Input: part model. Units: mm. Frame: model coordinates. Face numbers are marked on the shaded views. Round coordinates to 2 decimals unless told otherwise and drop trailing zeros. Order: outer loops, then holes, each group sorted by start corner. A loop starts at its lowest first (then second) coordinate and runs counter-clockwise, first axis right, second up. Notation, with made-up numbers: (-38, 61.25) - (10, 61.25) arc R33 ccw to (10, 92.25) - close; hole circle Ø9 at (-19.5, 40.5). An arc over 180 degrees is marked (long way). One line per item, written item: value. Start each with the question number.
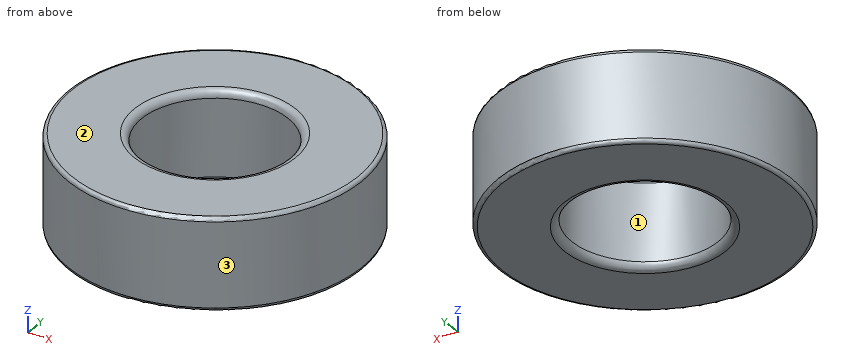
from build123d import *

# Parameters (mm, degrees)
BEARING_BOSS_EXTRUDE1_DEPTH      = 2.5
BEARING_BOSS_EXTRUDE1_DEPTH_BACK = 2.5
SKETCH1_R                        = 8
SKETCH1_R_2                      = 4
FILLET6_R                        = 0.2
FILLET7_R                        = 0.4


with BuildPart() as part:
    # Sketch1 → Bearing Boss-Extrude1 (new, two sides: drawn at the far end of the back side and taken through both)
    with BuildSketch(Plane.XY.offset(-BEARING_BOSS_EXTRUDE1_DEPTH_BACK)):
        Circle(SKETCH1_R)
        Circle(SKETCH1_R_2, mode=Mode.SUBTRACT)
    extrude(amount=BEARING_BOSS_EXTRUDE1_DEPTH + BEARING_BOSS_EXTRUDE1_DEPTH_BACK)

    # Fillet6
    fillet6_edges = [part.edges().sort_by_distance(p)[0] for p in [
        (-8, 0, -2.5),
        (-8, 0, 2.5),
    ]]
    fillet(fillet6_edges, radius=FILLET6_R)

    # Fillet7
    fillet7_edges = [part.edges().sort_by_distance(p)[0] for p in [
        (-4, 0, -2.5),
        (-4, 0, 2.5),
    ]]
    fillet(fillet7_edges, radius=FILLET7_R)


solid = part.part
Item 1: First-contact query: pin 1 Ø2 at (x, z) = (6, 1) entering from +Y (3 decimals); pin 2 Ø4 at (x, y) = (2, 1) entering from -Z. Flat tips, straight axial feed; report the tip coordinate or a pass-through.
Item 2: Pull-direction query (X, two-part tool) for the marked faces 1, 2 and 3; classes: released by +X, released by -X, zero draft, split by the parting line, or undercut.
Item 3: Line query: L1, parallel to Y at x = 0, z = 0.9; L2, parallel to X at y = 2.5, z = -1.6; L3, parallel to X at y = -0.75, z = -2.25. Output: solid intervals per line, ascending.
Item 4: Section query A-A on y = 0. Return loops of the section in (x, z), and give its area (3 significant figures).
Item 5: Section query C-C on z = -1.5. Return loops of the section in (x, y).
Geometry results:
1. pin 1: stops at y = 6.245
1. pin 2: stops at z = -2.46
2. face 1: undercut
2. face 2: zero draft
2. face 3: split by the parting line
3. L1: y = -8 to -4, 4 to 8
3. L2: x = -7.6 to -3.12, 3.12 to 7.6
3. L3: x = -7.96 to -3.96, 3.96 to 7.96
4. outline: (-8, -2.3) arc R0.2 ccw to (-7.8, -2.5) - (-4.4, -2.5) arc R0.4 ccw to (-4, -2.1) - (-4, 2.1) arc R0.4 ccw to (-4.4, 2.5) - (-7.8, 2.5) arc R0.2 ccw to (-8, 2.3) - close; (4, -2.1) arc R0.4 ccw to (4.4, -2.5) - (7.8, -2.5) arc R0.2 ccw to (8, -2.3) - (8, 2.3) arc R0.2 ccw to (7.8, 2.5) - (4.4, 2.5) arc R0.4 ccw to (4, 2.1) - close
4. area: 39.8 mm^2
5. outline: circle Ø16 at (0, 0); hole circle Ø8 at (0, 0)
